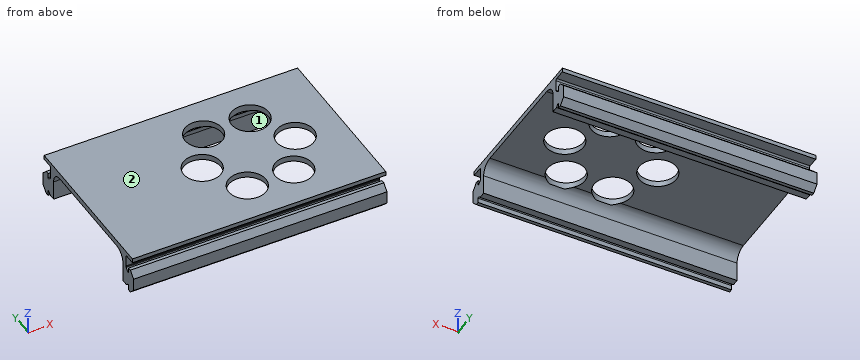
Autodesk Fusion 360 part; units mm, degrees
sketch "Sketch1" plane through (0, 0, 0) normal (1, 0, 0) x (0, 1, 0)
  line L0 (36.1, 2.8393) -> (36.1, 0.1999) construction
  line L1 (29.9076, 4.5417) -> (29.928, 4.4966)
  line L2 (-31.8, -5.5) -> (-31.8, -3.2628) construction
  line L3 (-36.1, 2.8393) -> (-36.1, 0.1999) construction
  line L4 (30.0626, 4.563) -> (30.0813, 4.5279) construction
  line L5 (31.4586, -3.1214) -> (30.1778, -4.4022) construction
  arc A0 (-31.3525, -3.0154) -> (-31.95, -3.2628) centre (-31.6, -3.2628) ccw
  line L6 (30.0462, 4.5991) -> (30.0626, 4.563) construction
  line L7 (30.1023, 4.4942) -> (30.1254, 4.4619) construction
  arc A1 (31.8, -3.2628) -> (31.4586, -3.1214) centre (31.6, -3.2628) ccw construction
  line L8 (30.0322, 4.6363) -> (30.0462, 4.5991) construction
  line L9 (31.8, -5.5) -> (31.8, -3.2628) construction
  line L10 (-31.95, -5.35) -> (-31.95, -3.2628)
  line L11 (-31.8, -5.5) -> (-31.8, -3.2628) construction
  line L12 (35.15, 10) -> (31.5, 10) construction
  line L13 (29.9514, 4.4529) -> (29.9775, 4.4108)
  arc A2 (-31.4586, -3.1214) -> (-31.8, -3.2628) centre (-31.6, -3.2628) ccw construction
  line L14 (31.95, -5.35) -> (31.95, -3.2628)
  line L15 (-33.4393, -5.5) -> (-31.8, -5.5) construction
  line L16 (33.4393, -5.5) -> (31.8, -5.5) construction
  line L17 (31.3525, -3.0154) -> (30.3679, -4)
  line L18 (29.8757, 4.6355) -> (29.8901, 4.5881)
  line L19 (29.8901, 4.5881) -> (29.9076, 4.5417)
  line L20 (-33.4393, -5.5) -> (-31.8, -5.5) construction
  arc A3 (-31.4586, -3.1214) -> (-31.8, -3.2628) centre (-31.6, -3.2628) ccw construction
  line L21 (35.15, 10) -> (31.5, 10) construction
  line L22 (-33.3772, -5.35) -> (-31.95, -5.35)
  line L23 (33.3772, 5.35) -> (35.95, 2.7772)
  line L24 (36.1, 2.8393) -> (36.1, 0.1999) construction
  line L25 (-31.3525, -3.0154) -> (-30.3679, -4)
  arc A4 (31.95, -3.2628) -> (31.3525, -3.0154) centre (31.6, -3.2628) ccw
  line L26 (33.4393, -5.5) -> (31.8, -5.5) construction
  line L27 (35.95, 2.7772) -> (35.95, 0.1377)
  arc A5 (31.8, -3.2628) -> (31.4586, -3.1214) centre (31.6, -3.2628) ccw construction
  line L28 (31.4586, -3.1214) -> (30.1778, -4.4022) construction
  line L29 (33.3772, -5.35) -> (31.95, -5.35)
  line L30 (31.8, -5.5) -> (31.8, -3.2628) construction
  line L31 (-29.9076, 4.5417) -> (-29.928, 4.4966)
  line L32 (-30.0626, 4.563) -> (-30.0813, 4.5279) construction
  line L33 (-36.1, 0.1999) -> (-36.2999, 0) construction
  line L34 (-30.0064, 4.3705) -> (-30.0378, 4.3322)
  line L35 (36.1, -0.1999) -> (36.1, -2.8393) construction
  line L36 (-30.1023, 4.4942) -> (-30.1254, 4.4619) construction
  line L37 (-30.0813, 4.5279) -> (-30.1023, 4.4942) construction
  line L38 (35.95, -0.1377) -> (35.95, -2.7772)
  line L39 (-29.8901, 4.5881) -> (-29.9076, 4.5417)
  line L40 (30.0117, 4.713) -> (30.0207, 4.6743) construction
  line L41 (-36.1, -0.1999) -> (-36.1, -2.8393) construction
  circle A6 centre (-40, 0) radius 2.1 construction
  line L42 (-30.0462, 4.5991) -> (-30.0626, 4.563) construction
  line L43 (30.0052, 4.7522) -> (30.0117, 4.713) construction
  line L44 (30.1023, 4.4942) -> (30.1254, 4.4619) construction
  line L45 (-30.0462, 4.5991) -> (-30.0626, 4.563) construction
  line L46 (30.0462, 4.5991) -> (30.0626, 4.563) construction
  line L47 (30.1254, 4.4619) -> (30.1506, 4.4312) construction
  line L48 (-36.1, 0.1999) -> (-36.2999, 0) construction
  line L49 (30.0813, 4.5279) -> (30.1023, 4.4942) construction
  line L50 (30.0626, 4.563) -> (30.0813, 4.5279) construction
  line L51 (-30.0813, 4.5279) -> (-30.1023, 4.4942) construction
  line L52 (29.9775, 4.4108) -> (30.0064, 4.3705)
  line L53 (-30.0626, 4.563) -> (-30.0813, 4.5279) construction
  line L54 (-36.2999, 0) -> (-36.1, -0.1999) construction
  line L55 (30.0378, 4.3322) -> (30.07, 4.2979)
  line L56 (30.0322, 4.6363) -> (30.0462, 4.5991) construction
  line L57 (30.0064, 4.3705) -> (30.0378, 4.3322)
  line L58 (-29.9775, 4.4108) -> (-30.0064, 4.3705)
  line L59 (-36.1, -0.1999) -> (-36.1, -2.8393) construction
  line L60 (-35.95, -0.1377) -> (-35.95, -2.7772)
  line L61 (-30.0378, 4.3322) -> (-30.07, 4.2979)
  line L62 (-36.2999, 0) -> (-36.1, -0.1999) construction
  line L63 (30.0813, 4.5279) -> (30.1023, 4.4942) construction
  line L64 (29.928, 4.4966) -> (29.9514, 4.4529)
  line L65 (-30.1254, 4.4619) -> (-30.1506, 4.4312) construction
  line L66 (-30.1254, 4.4619) -> (-30.1506, 4.4312) construction
  line L67 (30.1254, 4.4619) -> (30.1506, 4.4312) construction
  line L68 (-30.1023, 4.4942) -> (-30.1254, 4.4619) construction
  line L69 (36.1, 0.1999) -> (36.2999, 0) construction
  line L70 (-29.9514, 4.4529) -> (-29.9775, 4.4108)
  line L71 (30.0117, 4.713) -> (30.0207, 4.6743) construction
  line L72 (-29.928, 4.4966) -> (-29.9514, 4.4529)
  line L73 (29.8564, 4.7326) -> (29.8645, 4.6837)
  line L74 (30.0013, 4.7917) -> (30.0052, 4.7522) construction
  line L75 (-30.0322, 4.6363) -> (-30.0462, 4.5991) construction
  line L76 (-29.8757, 4.6355) -> (-29.8901, 4.5881)
  line L77 (30.07, 4.2979) -> (31.3525, 3.0154)
  line L78 (36.1, -0.1999) -> (36.1, -2.8393) construction
  circle A7 centre (40, 0) radius 2.1 construction
  line L79 (30.1506, 4.4312) -> (30.1778, 4.4022) construction
  circle A8 centre (40, 0) radius 2.1 construction
  line L80 (-35.15, 10) -> (-31.5, 10) construction
  line L81 (-30.0207, 4.6743) -> (-30.0322, 4.6363) construction
  line L82 (30.1506, 4.4312) -> (30.1778, 4.4022) construction
  line L83 (-29.8515, 4.7819) -> (-29.8564, 4.7326)
  line L84 (-30.0052, 4.7522) -> (-30.0117, 4.713) construction
  line L85 (-29.8645, 4.6837) -> (-29.8757, 4.6355)
  line L86 (36.1, 0.1999) -> (36.2999, 0) construction
  line L87 (-35, 10.15) -> (-31.5, 10.15)
  line L88 (36.2999, 0) -> (36.1, -0.1999) construction
  line L89 (30.0207, 4.6743) -> (30.0322, 4.6363) construction
  line L90 (-30.0052, 4.7522) -> (-30.0117, 4.713) construction
  line L91 (30.0207, 4.6743) -> (30.0322, 4.6363) construction
  line L92 (29.8645, 4.6837) -> (29.8757, 4.6355)
  line L93 (-35.95, -2.7772) -> (-33.3772, -5.35)
  line L94 (-36.1, -2.8393) -> (-33.4393, -5.5) construction
  line L95 (30.0013, 4.7917) -> (30.0052, 4.7522) construction
  line L96 (33.4393, 5.5) -> (36.1, 2.8393) construction
  line L97 (-30.0013, 4.7917) -> (-30.0052, 4.7522) construction
  line L98 (-30.0013, 4.7917) -> (-30.0052, 4.7522) construction
  line L99 (-30.0117, 4.713) -> (-30.0207, 4.6743) construction
  line L100 (30.1778, 4.4022) -> (31.4586, 3.1214) construction
  line L101 (30.0052, 4.7522) -> (30.0117, 4.713) construction
  line L102 (36.1, -2.8393) -> (33.4393, -5.5) construction
  line L103 (30.1778, 4.4022) -> (31.4586, 3.1214) construction
  line L104 (-30.0117, 4.713) -> (-30.0207, 4.6743) construction
  line L105 (-33.4393, 5.5) -> (-36.1, 2.8393) construction
  line L106 (-29.8564, 4.7326) -> (-29.8645, 4.6837)
  line L107 (36.1, -2.8393) -> (33.4393, -5.5) construction
  line L108 (-33.3772, 5.35) -> (-35.95, 2.7772)
  arc A9 (31.4586, 3.1214) -> (31.8, 3.2628) centre (31.6, 3.2628) ccw construction
  line L109 (29.8515, 4.7819) -> (29.8564, 4.7326)
  line L110 (36.2999, 0) -> (36.1, -0.1999) construction
  line L111 (-36.1, -2.8393) -> (-33.4393, -5.5) construction
  line L112 (-30.0207, 4.6743) -> (-30.0322, 4.6363) construction
  arc A10 (31.4586, 3.1214) -> (31.8, 3.2628) centre (31.6, 3.2628) ccw construction
  arc A11 (31.3525, 3.0154) -> (31.95, 3.2628) centre (31.6, 3.2628) ccw
  line L113 (35.95, -2.7772) -> (33.3772, -5.35)
  line L114 (33.4393, 5.5) -> (36.1, 2.8393) construction
  line L115 (35, 10.15) -> (31.5, 10.15)
  circle A12 centre (-40, 0) radius 2.1 construction
  line L116 (-30.0322, 4.6363) -> (-30.0462, 4.5991) construction
  line L117 (-31.95, 5.35) -> (-33.3772, 5.35)
  line L118 (30, 4.8314) -> (30.0013, 4.7917) construction
  line L119 (29.85, 4.829) -> (29.8515, 4.7819)
  line L120 (-30.1778, 4.4022) -> (-31.4586, 3.1214) construction
  line L121 (31.8, 5.5) -> (33.4393, 5.5) construction
  line L122 (-35.2083, 9.9987) -> (-35.15, 10) construction
  line L123 (-30, 4.8314) -> (-30.0013, 4.7917) construction
  line L124 (-35.2083, 9.9987) -> (-35.15, 10) construction
  arc A13 (30.5, 10) -> (30, 9.5) centre (30.5, 9.5) ccw construction
  line L125 (-31.95, 3.2628) -> (-31.95, 5.35)
  line L126 (-29.85, 4.829) -> (-29.8515, 4.7819)
  line L127 (30, 9.5) -> (30, 8.5) construction
  arc A14 (30.5, 10.15) -> (29.85, 9.5) centre (30.5, 9.5) ccw
  line L128 (30, 9.5) -> (30, 8.5) construction
  line L129 (31.95, 3.2628) -> (31.95, 5.35)
  arc A15 (-31.8, 3.2628) -> (-31.4586, 3.1214) centre (-31.6, 3.2628) ccw construction
  arc A16 (-31.8, 3.2628) -> (-31.4586, 3.1214) centre (-31.6, 3.2628) ccw construction
  line L130 (31.95, 5.35) -> (33.3772, 5.35)
  line L131 (-30.07, 4.2979) -> (-31.3525, 3.0154)
  arc A17 (-31.95, 3.2628) -> (-31.3525, 3.0154) centre (-31.6, 3.2628) ccw
  line L132 (-33.4393, 5.5) -> (-36.1, 2.8393) construction
  line L133 (-30.1506, 4.4312) -> (-30.1778, 4.4022) construction
  line L134 (29.85, 9.5) -> (29.85, 8.5)
  line L135 (-30.1778, 4.4022) -> (-31.4586, 3.1214) construction
  line L136 (31.5, 10) -> (30.5, 10) construction
  line L137 (30, 8.5) -> (30, 4.8314) construction
  line L138 (-31.5, 10) -> (-30.5, 10) construction
  line L139 (31.8, 3.2628) -> (31.8, 5.5) construction
  line L140 (30, 4.8314) -> (30.0013, 4.7917) construction
  line L141 (-31.5, 10.15) -> (-30.5, 10.15)
  arc A18 (30.5, 10) -> (30, 9.5) centre (30.5, 9.5) ccw construction
  arc A19 (-30, 9.5) -> (-30.5, 10) centre (-30.5, 9.5) ccw construction
  line L142 (-30.1506, 4.4312) -> (-30.1778, 4.4022) construction
  line L143 (31.8, 5.5) -> (33.4393, 5.5) construction
  line L144 (-35.15, 10) -> (-31.5, 10) construction
  line L145 (31.8, 3.2628) -> (31.8, 5.5) construction
  line L146 (30, 8.5) -> (30, 4.8314) construction
  line L147 (-30, 4.8314) -> (-30.0013, 4.7917) construction
  line L148 (29.85, 8.5) -> (29.85, 4.829)
  line L149 (-30, 9.5) -> (-30, 8.5) construction
  line L150 (-29.85, 9.5) -> (-29.85, 8.5)
  arc A20 (-29.85, 9.5) -> (-30.5, 10.15) centre (-30.5, 9.5) ccw
  line L151 (31.5, 10) -> (30.5, 10) construction
  line L152 (-29.85, 8.5) -> (-29.85, 4.829)
  line L153 (-31.8, 5.5) -> (-33.4393, 5.5) construction
  line L154 (-31.8, 3.2628) -> (-31.8, 5.5) construction
  arc A21 (-30, 9.5) -> (-30.5, 10) centre (-30.5, 9.5) ccw construction
  line L155 (-31.8, 5.5) -> (-33.4393, 5.5) construction
  line L156 (-31.5, 10) -> (-30.5, 10) construction
  line L157 (-31.8, 3.2628) -> (-31.8, 5.5) construction
  line L158 (-30, 9.5) -> (-30, 8.5) construction
  line L159 (-30, 8.5) -> (-30, 4.8314) construction
  line L160 (31.5, 10.15) -> (30.5, 10.15)
  line L161 (-30, 8.5) -> (-30, 4.8314) construction
  line L162 (0, 15) -> (0, -15) construction
  line L163 (-35.95, 2.7772) -> (-35.95, 0.1377)
  line L164 (-36.1, 2.8393) -> (-36.1, 0.1999) construction
  line L165 (35, 10.15) -> (35, 12)
  line L166 (35, 12) -> (-35, 12)
  line L167 (-35, 12) -> (-35, 10.15)
  line L168 (30.3679, -4) -> (27.5, -4)
  line L169 (27.5, -4) -> (27.5, 9.5)
  line L170 (27.5, 9.5) -> (-27.5, 9.5)
  line L171 (-27.5, 9.5) -> (-27.5, -4)
  line L172 (-27.5, -4) -> (-30.3679, -4)
  line L173 (35.95, 0.1377) -> (35.95, -0.1377)
  line L174 (-35.95, 0.1377) -> (-35.95, -0.1377)
  dimension "d1" = 16
extrude "Extrude1" add sketch "Sketch1" along normal blind 109
fillet "Fillet1" radius 5 2 edges at (54.5, -27.5, 9.5) (54.5, 27.5, 9.5)
sketch "Sketch2" plane through (0, 0, 12) normal (0, 0, 1) x (-1, 0, 0)
  line L0 (0, -35) -> (0, 35)
  line L1 (0, 35) -> (-109, 35)
  line L2 (-109, 35) -> (-109, -35)
  line L3 (-109, -35) -> (0, -35)
  line L4 (-109, 0) -> (0, 0) construction
  line L5 (-69, 0) -> (-89, 0) construction
  circle A0 centre (-89, 0) radius 8
  circle A1 centre (-79, -17.3205) radius 8
  circle A2 centre (-59, -17.3205) radius 8
  circle A3 centre (-49, 0) radius 8
  circle A4 centre (-59, 17.3205) radius 8
  circle A5 centre (-79, 17.3205) radius 8
  dimension "d11" = 20
  dimension "d12" = 16
  dimension "d14" = 360
extrude "Extrude2" cut sketch "Sketch2" against normal blind 3 contours A0 | A1 | A2 | A3 | A4 | A5
Design review of the part built by this model. Coordinates are the model's own, in mm. Face numbers are marked on the shaded views. Give positions to 0.01 mm unless a question says otherwise; leave off trailing zeros. Write each loop counter-clockwise with the first axis right and the second up, starting at its lowest first coordinate (ties: lowest second). Pieces come first, ordered by that corner, then holes.
(1) Wall thickness on line 1 along Y through (x, z) = (79, 9.65); line 2 along Y through (x, z) = (59, 10.95); line 3 along X through (y, z) = (0, 10.7): over which ranges is each line inside the solid? List them lowest first.
Checked values:
line 1: y = -29.87 to -25.32, -9.32 to 9.32, 25.32 to 29.87
line 2: y = -35 to -25.32, -9.32 to 9.32, 25.32 to 35
line 3: x = 0 to 41, 57 to 81, 97 to 109
(2) Mouldability with a two-part tool opening along Y and no side actions: class the marked faces 1 and 2 as +Y half, -Y half, draft (parallel to the pull), parting line (faces both ways), or undercut.
Checked values:
face 1: undercut
face 2: draft
(3) Add section C-C (x = 79). Give the number of separate pieces and of enclosed holes in the cut face, and give its area (3 significant figures).
Checked values:
separate pieces: 3
enclosed holes: 0
area: 263 mm2
(4) Add section A-A (z = 1). Give the boundary of the cut face in (x, y).
Checked values:
outline: (0, -35.95) - (109, -35.95) - (109, -27.5) - (0, -27.5) - close; (0, 27.5) - (109, 27.5) - (109, 35.95) - (0, 35.95) - close
(5) Clearance check with flat-ended pins moving along their axes: pin 1 Ø0.9 at (x, z) = (27.5, 11.5) entering from -Y; pin 2 Ø1.5 at (x, y) = (84.5, -28) entering from -Z; pin 3 Ø5 at (x, z) = (35, 7) entering from +Y. State where each tip first meets the part, or that it passes through.
Checked values:
pin 1: stops at y = -35
pin 2: stops at z = -4
pin 3: stops at y = 34.23
(6) Add section D-D (y = -18.5). Give the boundary of the cut face in (x, z), and give its area (3 significant figures).
Checked values:
outline: (0, 9.5) - (51.09, 9.5) - (51.09, 12) - (0, 12) - close; (66.91, 9.5) - (71.09, 9.5) - (71.09, 12) - (66.91, 12) - close; (86.91, 9.5) - (109, 9.5) - (109, 12) - (86.91, 12) - close
area: 193 mm2
(7) Add section B-B (y = 0). Give the boundary of the cut face in (x, z), and give its area (4 significant figures).
Checked values:
outline: (0, 9.5) - (41, 9.5) - (41, 12) - (0, 12) - close; (57, 9.5) - (81, 9.5) - (81, 12) - (57, 12) - close; (97, 9.5) - (109, 9.5) - (109, 12) - (97, 12) - close
area: 192.5 mm2
